Source: CAD feature listing. Evaluate the final solid. Frame: model axes, mm. A direction names the side the tool comes from. Coordinates: 2 decimals unless noted, no trailing zeros. Write each loop counter-clockwise with the first axis right and the second up, starting at its lowest first coordinate (ties: lowest second). Pieces come first, ordered by that corner, then holes. Notation, with made-up numbers: (55.5, 83) - (96.5, 83) arc R21 ccw to (96.5, 98) - close; hole circle Ø2 at (64, 58). An arc over 180 degrees is marked (long way). One line per item, written item: value.
from build123d import *

# Parameters (mm, degrees)
BOSS_EXTRUDE1_DEPTH = 3
FILLET1_R           = 5
FILLET2_R           = 2
FILLET3_R           = 7
FILLET4_R           = 2
FILLET5_R           = 5


with BuildPart() as part:
    # Sketch1 → Boss-Extrude1 (new body)
    with BuildSketch(Plane(origin=(0, 0, 0), x_dir=(1, 0, 0), z_dir=(0, 1, 0))):
        with BuildLine():
            Line((0, 33.06), (0, 0))
            Line((0, 0), (14.8, 0))
            Line((14.8, 0), (14.8, 9.13))
            ThreePointArc((14.8, 9.13), (16.3, 10.63), (17.8, 9.13))
            Line((17.8, 9.13), (17.8, 0))
            Line((17.8, 0), (28.82, 0))
            Line((28.82, 0), (40.93, 25.6))
            Line((40.93, 25.6), (23.039915269, 25.6))
            ThreePointArc((23.039915269, 25.6), (21.54, 27.084056775), (23.00803062, 28.599661085))
            Line((23.00803062, 28.599661085), (30.66, 28.762351413))
            Line((30.66, 28.762351413), (46.79, 78.9))
            Line((46.79, 78.9), (34.22, 83.484702826))
            Line((34.22, 83.484702826), (20.171354305, 41.75831525))
            ThreePointArc((20.171354305, 41.75831525), (12.025034014, 32.911797705), (0, 33.06))
        make_face()
    extrude(amount=BOSS_EXTRUDE1_DEPTH)

    # Fillet1
    fillet1_edges = [part.edges().sort_by_distance(p)[0] for p in [
        (40.93, 1.5, -25.6),
    ]]
    fillet(fillet1_edges, radius=FILLET1_R)

    # Fillet2
    fillet2_edges = [part.edges().sort_by_distance(p)[0] for p in [
        (0, 1.5, -33.06),
    ]]
    fillet(fillet2_edges, radius=FILLET2_R)

    # Fillet3
    fillet3_edges = [part.edges().sort_by_distance(p)[0] for p in [
        (34.22, 1.5, -83.484702826),
    ]]
    fillet(fillet3_edges, radius=FILLET3_R)

    # Fillet4
    fillet4_edges = [part.edges().sort_by_distance(p)[0] for p in [
        (0, 1.5, 0),
        (46.79, 1.5, -78.9),
    ]]
    fillet(fillet4_edges, radius=FILLET4_R)

    # Fillet5
    fillet5_edges = [part.edges().sort_by_distance(p)[0] for p in [
        (28.82, 1.5, 0),
    ]]
    fillet(fillet5_edges, radius=FILLET5_R)


solid = part.part
1) Material intervals for line 1 (X direction, y = 2.7, z = -4.5); line 2 (Z direction, x = 5.5, y = 1.05); line 3 (X direction, y = 2.95, z = -21), sorted ascending.
Values found:
line 1: 0 to 14.8, 17.8 to 30.95
line 2: -31.72 to 0
line 3: 0 to 38.02
2) Section query C-C on z = -27.1. Output: boundary loops of the cut face in (x, y).
Values found:
outline: (0, 0) - (21.54, 0) - (21.54, 3) - (0, 3) - close
3) Contact query for flat-ended pins moving along their axis: P1, Ø3, axis at x = 14.5, z = -36.5, coming from the -Y side; P2, Ø0.9, axis at y = 1, z = -6, coming from the +X side. Output: stop coordinate, or through.
Values found:
P1: through
P2: x = 31.87
4) Draft query along Z for faces 4 (the flat face through (26.133, 1.479, -59.465)), 5 (the flat face through (28, 1, -25.6)), 6 (the cylindrical face through (46.084, 1.521, -78.578)), 7 (the flat face through (23, 3, -32)). Return one class per face: released by +Z, released by -Z, zero draft, split by the parting line, or undercut.
Values found:
face 4: released by -Z
face 5: undercut
face 6: split by the parting line
face 7: zero draft
5) Reachability of faces 1 (the flat face through (38.322, 1.479, -52.577)), 2 (the flat face through (23, 0, -32)), 3 (the flat face through (17.8, 1, -5)) from +Z, -Z, +X, -X, +Y, -Y: full face, straight path, thin tool, end or side. Return the list, or none.
Values found:
face 1: +X, +Y, -Y
face 2: +Z, -Z, +X, -X, -Y
face 3: +Z, +Y, -Y
6) Section query D-D on x = 12. Output: boundary loops of the cut face in (y, z), then the cut area to 3 significant figures.
Values found:
outline: (0, -32.9) - (3, -32.9) - (3, 0) - (0, 0) - close
area: 98.7 mm2
7) Section query B-B on y = 2.5. Output: boundary loops of the cut face in (x, z).
Values found:
outline: (0, -30.23) arc R2 ccw to (2.5, -32.17) arc R14.76 cw to (20.17, -41.76) - (31.93, -76.68) arc R7 ccw to (40.96, -81.03) - (44.98, -79.56) arc R2 ccw to (46.2, -77.07) - (30.66, -28.76) - (23.01, -28.6) arc R1.5 cw to (23.04, -25.6) - (33.03, -25.6) arc R5 ccw to (37.55, -18.46) - (30.17, -2.86) arc R5 ccw to (25.65, 0) - (17.8, 0) - (17.8, -9.13) arc R1.5 cw to (14.8, -9.13) - (14.8, 0) - (2, 0) arc R2 ccw to (0, -2) - close
8) Section query A-A on z = -4.5. Output: boundary loops of the cut face in (x, y), then the cut area to 3 significant figures.
Values found:
outline: (0, 0) - (14.8, 0) - (14.8, 3) - (0, 3) - close; (17.8, 0) - (30.95, 0) - (30.95, 3) - (17.8, 3) - close
area: 83.8 mm2
